The listing builds one solid part. Answer for the finished solid, in the listing's coordinates (mm). A direction names the side the tool comes from. Give positions to 0.01 mm unless a question says otherwise; leave off trailing zeros. Order: outer loops, then holes, each group sorted by start corner. A loop starts at its lowest first (then second) coordinate and runs counter-clockwise, first axis right, second up. Notation, with made-up numbers: (28, 43) - (43, 43) arc R16 cw to (43, 68) - close; hole circle Ø11 at (-27.5, -25). An arc over 180 degrees is marked (long way). Answer as CSV lines item,"result". Start each with the question number.
1. Which of the six approach directions +Z, -Z, +X, -X, +Y, -Y give full straight-line access (tool end or side, diameter ignored) to faces 1 (the cylindrical face through (36.605, 0.42, 11.266)), 2 (the cylindrical face through (-30.53, 0.42, 11.96))?
2. Section C-C on x = -19.5 is taken. Give the vertices of the cut face in (y, z).
3. Flat-ended cylindrical pins translate along their axes: pin 1 (1 mm diameter, centred on x = 23, z = -16.5, fed in from +Y); pin 2 (1.5 mm diameter, centred on x = 29, z = -4, fed in from -Y); pin 3 (1.5 mm diameter, centred on x = -10.5, z = -11, fed in from -Y); pin 4 (5 mm diameter, centred on x = -9, z = -3, fed in from -Y). Find the tip coordinate at first contact, or state that the pin passes through.
4. Consider line 1 along X through (y, z) = (4.5, 0); line 2 along X through (y, z) = (-22.5, -0.5); line 3 along Z through (x, y) = (11, 17). Determine where each line is inside the solid, lowest interval first. Write a range as [from, to].
5. Section A-A on z = -3 is taken. Give the vertices of the cut face in (x, y).
6. Determine the mould class of faces 3 (the cylindrical face through (30.53, 0.42, 11.96)), 4 (the cylindrical face through (-36.68, 0.42, 11.19)), 5 (the flat face through (-31, 30, 5)) for opening direction X: +X half, -X half, draft (parallel to the pull), parting line (faces both ways), or undercut.
7. Section B-B on y = 23.5 is taken. Give the vertices of the cut face in (x, z), and give its area (3 significant figures).
8. Section D-D on y = 15.5 is taken. Give the vertices of the cut face in (x, z), and give its area (3 significant figures).
from build123d import *

# Parameters (mm, degrees)
F1_DEPTH      = 38.1
F1_DEPTH_BACK = 38.1
F3_DEPTH      = 30.48
F3_DEPTH_BACK = 30.48
F4_T1_DEPTH   = 85
F4_T3_DEPTH   = 75.73883536


# Not quite as in the source:
# - a fillet or chamfer that OpenCascade refuses, or shapes differently, is made with other operations: its cross-section is extruded or revolved along the edge and cut away or added


with BuildPart() as f1:
    # F0 (on Right) → F1 (new body, two sides)
    with BuildSketch(Plane.YZ) as f1_sk:
        with BuildLine():
            Line((-30, 12.7), (-30, 0))
            ThreePointArc((-30, 0), (0, -22.5972709807), (30, 0))
            Line((30, 0), (30, 12.7))
            Line((30, 12.7), (-30, 12.7))
        make_face()
    extrude(amount=F1_DEPTH)
    extrude(f1_sk.sketch, amount=-F1_DEPTH_BACK)

    # F2 (on Front) → F3 (cut, two sides)
    with BuildSketch(Plane.XZ) as f3_sk:
        with BuildLine():
            Line((30, 12.7), (-30, 12.7))
            ThreePointArc((-30, 12.7), (0, -7.177446186), (30, 12.7))
        make_face()
    extrude(amount=-F3_DEPTH, mode=Mode.SUBTRACT)
    extrude(f3_sk.sketch, amount=F3_DEPTH_BACK, mode=Mode.SUBTRACT)

    # F4: fillet of radius 5 on 4 edges, made by hand

    # F4_s2 → F4_t1 (cut)
    with BuildSketch(Plane.XZ.offset(-42.5)):
        with BuildLine():
            ThreePointArc((-38.1, 7.7), (-36.6355339059, 11.2355339059), (-33.1, 12.7))
            Line((-33.1, 12.7), (-38.1, 12.7))
            Line((-38.1, 12.7), (-38.1, 7.7))
        make_face()
        with BuildLine():
            ThreePointArc((33.1, 12.7), (36.6355339059, 11.2355339059), (38.1, 7.7))
            Line((38.1, 7.7), (38.1, 12.7))
            Line((38.1, 12.7), (33.1, 12.7))
        make_face()
    extrude(amount=F4_T1_DEPTH, mode=Mode.SUBTRACT)

    # F4_s4 → F4_t3 (cut)
    with BuildSketch(Plane.XZ.offset(-37.86941768)):
        with BuildLine():
            ThreePointArc((-28.7371736927, 10.0551360984), (-30.5763550564, 11.988104505), (-33.147767072, 12.7))
            Line((-33.147767072, 12.7), (-30, 12.7))
            ThreePointArc((-30, 12.7), (-29.3983455251, 11.3633593626), (-28.7371736927, 10.0551360984))
        make_face()
        with BuildLine():
            ThreePointArc((28.7371736927, 10.0551360984), (30.5763550564, 11.988104505), (33.147767072, 12.7))
            Line((33.147767072, 12.7), (30, 12.7))
            ThreePointArc((30, 12.7), (29.3983455251, 11.3633593626), (28.7371736927, 10.0551360984))
        make_face()
    extrude(amount=F4_T3_DEPTH, mode=Mode.SUBTRACT)


solid = f1.part
Checks:
1,face 1,"+Z, +X, +Y, -Y"
1,face 2,"+Z, +Y, -Y"
2,outline,"(-29.79, -0.7) arc R31.21 ccw to (29.79, -0.7) - close"
3,pin 1,"stops at y = 19.19"
3,pin 2,"stops at y = -28.87"
3,pin 3,"stops at y = -24.87"
3,pin 4,"passes through"
4,line 1,"x = [-38.1, -20.4], [20.4, 38.1]"
4,line 2,"x = [-38.1, -19.76], [19.76, 38.1]"
4,line 3,"z = [-17.56, -5.26]"
5,outline,"(-38.1, -28.97) - (-15.96, -28.97) - (-15.96, 28.97) - (-38.1, 28.97) - close; (15.96, -28.97) - (38.1, -28.97) - (38.1, 28.97) - (15.96, 28.97) - close"
6,face 3,"undercut"
6,face 4,"-X half"
6,face 5,"draft"
7,outline,"(-38.1, -11.93) - (38.1, -11.93) - (38.1, 7.7) arc R5 ccw to (33.12, 12.7) arc R5 ccw to (28.74, 10.06) arc R32.58 cw to (-28.74, 10.06) arc R5 ccw to (-33.12, 12.7) arc R5 ccw to (-38.1, 7.7) - close"
7,area,"1,000 mm²"
8,outline,"(-38.1, -18.48) - (38.1, -18.48) - (38.1, 7.7) arc R5 ccw to (33.12, 12.7) arc R5 ccw to (28.74, 10.06) arc R32.58 cw to (-28.74, 10.06) arc R5 ccw to (-33.12, 12.7) arc R5 ccw to (-38.1, 7.7) - close"
8,area,"1,500 mm²"
